from build123d import *

# Parameters (mm, degrees)
SKETCH1_W           = 63
SKETCH1_H           = 63
BOSS_EXTRUDE1_DEPTH = 4
SKETCH2_W           = 3
SKETCH2_H           = 6
CUT_EXTRUDE1_DEPTH  = 4
SKETCH3_W           = 9
SKETCH3_H           = 4
BOSS_EXTRUDE2_DEPTH = 3
SKETCH4_W           = 9
SKETCH4_H           = 4
BOSS_EXTRUDE3_DEPTH = 3
SKETCH5_W           = 26
SKETCH5_H           = 26
CUT_EXTRUDE2_DEPTH  = 4
SKETCH6_W           = 13
SKETCH6_H           = 10.5
CUT_EXTRUDE3_DEPTH  = 4
SKETCH8_W           = 6.5
SKETCH8_H           = 6
CUT_EXTRUDE4_DEPTH  = 1.5


with BuildPart() as part:
    # Sketch1 → Boss-Extrude1 (new body)
    with BuildSketch(Plane(origin=(0, 0, 0), x_dir=(1, 0, 0), z_dir=(0, 1, 0))):
        with Locations((31.5, 31.5)):
            Rectangle(SKETCH1_W, SKETCH1_H)
    extrude(amount=BOSS_EXTRUDE1_DEPTH)

    # Sketch2 → Cut-Extrude1 (cut)
    with BuildSketch(Plane(origin=(0, 4, 0), x_dir=(1, 0, 0), z_dir=(0, 1, 0))):
        with Locations((4.5, 3)):
            Rectangle(SKETCH2_W, SKETCH2_H)
        with Locations((58.5, 3)):
            Rectangle(SKETCH2_W, SKETCH2_H)
        with Locations((58.5, 60)):
            Rectangle(SKETCH2_W, SKETCH2_H)
        with Locations((4.5, 60)):
            Rectangle(SKETCH2_W, SKETCH2_H)
    extrude(amount=-CUT_EXTRUDE1_DEPTH, mode=Mode.SUBTRACT)

    # Sketch3 → Boss-Extrude2 (add)
    with BuildSketch(Plane.XY):
        with Locations((4.5, 2)):
            Rectangle(SKETCH3_W, SKETCH3_H)
        with Locations((58.5, 2)):
            Rectangle(SKETCH3_W, SKETCH3_H)
    extrude(amount=BOSS_EXTRUDE2_DEPTH)

    # Sketch4 → Boss-Extrude3 (add)
    with BuildSketch(Plane(origin=(0, 0, -63), x_dir=(-1, 0, 0), z_dir=(0, 0, -1))):
        with Locations((-4.5, 2)):
            Rectangle(SKETCH4_W, SKETCH4_H)
        with Locations((-58.5, 2)):
            Rectangle(SKETCH4_W, SKETCH4_H)
    extrude(amount=BOSS_EXTRUDE3_DEPTH)

    # Sketch5 → Cut-Extrude2 (cut)
    with BuildSketch(Plane(origin=(0, 4, 0), x_dir=(1, 0, 0), z_dir=(0, 1, 0))):
        with Locations((31.5, 31.5)):
            Rectangle(SKETCH5_W, SKETCH5_H)
    extrude(amount=-CUT_EXTRUDE2_DEPTH, mode=Mode.SUBTRACT)

    # Sketch6 → Cut-Extrude3 (cut)
    with BuildSketch(Plane(origin=(0, 4, 0), x_dir=(1, 0, 0), z_dir=(0, 1, 0))):
        with Locations((27, 57.75)):
            Rectangle(SKETCH6_W, SKETCH6_H)
    extrude(amount=-CUT_EXTRUDE3_DEPTH, mode=Mode.SUBTRACT)

    # Sketch8 → Cut-Extrude4 (cut)
    with BuildSketch(Plane.XZ):
        with Locations((41.032593784, -10)):
            Rectangle(SKETCH8_W, SKETCH8_H)
    extrude(amount=-CUT_EXTRUDE4_DEPTH, mode=Mode.SUBTRACT)


solid = part.part
Source: CAD feature listing. Evaluate the final solid. Frame: model axes, mm. A direction names the side the tool comes from. Coordinates: 2 decimals unless noted, no trailing zeros. Loops run counter-clockwise (first coordinate to the right, second up) from the corner with the lowest first, then second, coordinate; pieces in that order, holes last. Notation, with made-up numbers: (67.5, 28) - (87.5, 28) arc R24 ccw to (87.5, 50) - close; hole circle Ø7 at (-18.5, -39). An arc over 180 degrees is marked (long way). One line per item, written item: value. Start each with the question number.
1. Section D-D (y = 2.8). State how many separate pieces and enclosed holes the cut face has, and give its area (3 significant figures).
2. Section A-A (z = -31). Return the cut outline in (x, y), and give its area (3 significant figures).
3. Contact query for a flat-ended pin moving along its axis: P1, Ø1.5, axis at x = 11.5, y = 1.5, coming from the -Z side. Output: stop coordinate, or through.
4. Ray query, L1, parallel to X at y = 2.95, z = -57.5; L2, parallel to X at y = 1.65, z = -3; L3, parallel to X at y = 3.3, z = -38. Return the intervals inside material, ascending.
5. Set-up query: faces 4 (the flat face through (9, 2, -64)), 5 (the flat face through (9, 2, 1)), 6 (the flat face through (41, 1, -13)), 7 (the flat face through (57, 2, -60)). Return all of +Z, -Z, +X, -X, +Y, -Y with unobstructed straight access to the full face (end or side cutting, diameter ignored); none if empty.
6. Section C-C (x = 26.5). Return the cut outline in (y, z), and give its area (3 significant figures).
7. Section B-B (x = 43). Return the cut outline in (y, z), and give its area (3 significant figures).
8. Mould query, pull axis X, two halves, no side actions, for faces 1 (the flat face through (5, 2, -63)), 2 (the flat face through (63, 2, -31)), 3 (the flat face through (32, 4, -16)). Classes: pulls with the +X half, pulls with the -X half, needs draft (parallel to the pull), parting line crosses it, or undercut.
Verdict:
1. separate pieces: 1
1. enclosed holes: 5
1. area: 3,190 mm2
2. outline: (0, 0) - (18.5, 0) - (18.5, 4) - (0, 4) - close; (44.5, 0) - (63, 0) - (63, 4) - (44.5, 4) - close
2. area: 148 mm2
3. P1: stops at z = -63
4. L1: x = 0 to 3, 6 to 20.5, 33.5 to 57, 60 to 63
4. L2: x = 0 to 3, 6 to 57, 60 to 63
4. L3: x = 0 to 18.5, 44.5 to 63
5. face 4: -Z, +Y, -Y
5. face 5: +Z, +Y, -Y
5. face 6: -Y
5. face 7: +Y, -Y
6. outline: (0, -52.5) - (4, -52.5) - (4, -44.5) - (0, -44.5) - close; (0, -18.5) - (4, -18.5) - (4, 0) - (0, 0) - close
6. area: 106 mm2
7. outline: (0, -63) - (4, -63) - (4, -44.5) - (0, -44.5) - close; (0, -18.5) - (4, -18.5) - (4, 0) - (0, 0) - (0, -7) - (1.5, -7) - (1.5, -13) - (0, -13) - close
7. area: 139 mm2
8. face 1: undercut
8. face 2: pulls with the +X half
8. face 3: needs draft
